Check sheet for the modelled part. Datum: model origin and axes. Units: mm. A direction names the side the tool comes from. Give positions to 0.01 mm unless a question says otherwise; leave off trailing zeros. Loops run counter-clockwise (first coordinate to the right, second up) from the corner with the lowest first, then second, coordinate; pieces in that order, holes last. Notation, with made-up numbers: (6, 33) - (50, 33) arc R21 cw to (50, 48) - close; hole circle Ø7 at (42, 17.25). An arc over 180 degrees is marked (long way). Answer in a Markdown table with one row per item. Add a question column.
(1) Sectioned sample at A-A on y = 0. Enter the section's corners in (x, z) (3 decimals).
(2) Set-up check for faces 1 (the face through (1.802, 8.285, 5.723)), 2 (the face through (0.672, -7.454, -16.054)), 3 (the face through (-12.24, -6.25, 38.88)), 4 (the face through (26.971, -8.148, -35.175)): record each of +Z, -Z, +X, -X, +Y, -Y from which the full face is reachable in a straight line by a thin tool's end or side.
(3) Draft check along Z on faces 5 (the face through (4.5, 10.75, -4.5)), 6 (the face through (13.951, 10.562, -18.195)), 7 (the face through (-16.25, -7.45, -0.05)). Enter one of: released by +Z, released by -Z, zero draft, split by the parting line, or undercut.
(4) Go/stop test with flat-tipped pins: P1, Ø2, axis at x = 10, z = 0, coming from the +Y side; P2, Ø4, axis at y = -0.5, z = 6.5, coming from the -X side; P3, Ø2, axis at x = -15, z = 0, coming from the -Y side. Record where each tip stops, or that it passes through.
(5) Thickness scan on L1, parallel to X at y = 5.5, z = -17.5; L2, parallel to X at y = -9.5, z = 16; L3, parallel to X at y = -0.25, z = 25. Record the ranges inside material, lowest first.
from build123d import *

# Parameters (mm, degrees)
M3X0_5_TAPPED_HOLE1_D     = 2.5
M3X0_5_TAPPED_HOLE1_DEPTH = 6.5
M3X0_5_TAPPED_HOLE1_TIP   = 0.751075774
SKETCH4_R                 = 6
CUT_EXTRUDE1_DEPTH        = 5
M3X0_5_TAPPED_HOLE2_D     = 2.5
M3X0_5_TAPPED_HOLE2_DEPTH = 6.5
M3X0_5_TAPPED_HOLE2_TIP   = 0.751075774


with BuildPart() as part:
    # Sketch1 → Revolve1 (revolve)
    with BuildSketch(Plane.XY, mode=Mode.PRIVATE) as revolve1_sk:
        Polygon((0, -10.75), (0, 10.75), (-21.5, 10.75), (-44.325, 7.75), (-44.325, -6), (-40.7625, -6), (-40.7625, -6.5), (-44.325, -6.5), (-44.325, -9.75), (-35, -10.75), align=None)
    revolve(revolve1_sk.sketch.rotate(Axis((0, 0, 0), (0, -1, 0)), 270), axis=Axis((0, 0, 0), (0, -1, 0)))

    # M3x0.5 Tapped Hole1
    with Locations(Plane(origin=(0, 10.75, 0), x_dir=(1, 0, 0), z_dir=(0, 1, 0))):
        with Locations((0, 17.5), (0, 10), (17.5, 0), (10, 0), (0, -17.5), (0, -10), (-17.5, 0), (-10, 0)):
            Hole(M3X0_5_TAPPED_HOLE1_D / 2, depth=M3X0_5_TAPPED_HOLE1_DEPTH)
            with Locations((0, 0, -(M3X0_5_TAPPED_HOLE1_DEPTH + M3X0_5_TAPPED_HOLE1_TIP / 2))):  # 118° drill point
                Cone(0, M3X0_5_TAPPED_HOLE1_D / 2, M3X0_5_TAPPED_HOLE1_TIP, mode=Mode.SUBTRACT)

    # Sketch4 → Cut-Extrude1 (cut)
    with BuildSketch(Plane(origin=(0, 10.75, 0), x_dir=(1, 0, 0), z_dir=(0, 1, 0))):
        with Locations(Location((0, 0, 0), (0, 0, 270))):
            Circle(SKETCH4_R)
    extrude(amount=-CUT_EXTRUDE1_DEPTH, mode=Mode.SUBTRACT)

    # M3x0.5 Tapped Hole2
    with Locations(Plane(origin=(0, -10.75, 0), x_dir=(-1, 0, 0), z_dir=(0, -1, 0))):
        with Locations((0, 15), (15, 0), (0, -15), (-15, 0)):
            Hole(M3X0_5_TAPPED_HOLE2_D / 2, depth=M3X0_5_TAPPED_HOLE2_DEPTH)
            with Locations((0, 0, -(M3X0_5_TAPPED_HOLE2_DEPTH + M3X0_5_TAPPED_HOLE2_TIP / 2))):  # 118° drill point
                Cone(0, M3X0_5_TAPPED_HOLE2_D / 2, M3X0_5_TAPPED_HOLE2_TIP, mode=Mode.SUBTRACT)


solid = part.part
Reply:
| question | item | result |
|---|---|---|
| 1 | outline | circle Ø88.65 at (0, 0) |
| 2 | face 1 | +Y |
| 2 | face 2 | -Y |
| 2 | face 3 | none |
| 2 | face 4 | +Y, -Y |
| 3 | face 5 | zero draft |
| 3 | face 6 | split by the parting line |
| 3 | face 7 | undercut |
| 4 | P1 | y = 4.1 |
| 4 | P2 | x = -44.1 |
| 4 | P3 | y = -4.1 |
| 5 | L1 | -40.72 to -1.25, 1.25 to 40.72 |
| 5 | L2 | -41.34 to -0.75, 0.75 to 41.34 |
| 5 | L3 | -36.6 to 36.6 |
